Can you work these out from the model? Positions are in its coordinate system, mm. A direction names the side the tool comes from. Give positions to 0.01 mm unless a question says otherwise; leave off trailing zeros. Loops run counter-clockwise (first coordinate to the right, second up) from the corner with the lowest first, then second, coordinate; pieces in that order, holes last. Notation, with made-up numbers: (23.5, 59) -> (45.5, 59) arc R29 ccw to (45.5, 80) -> close; hole circle Ø4 at (86, 29). An arc over 180 degrees is marked (long way). Use CSV: the item, a comma, the result in double quotes.
from build123d import *

# Parameters (mm, degrees)
BOSS_EXTRUDE1_DEPTH      = 4.5
BOSS_EXTRUDE1_DEPTH_BACK = 4.5
SKETCH1_R                = 6.5
SKETCH1_R_2              = 4.5
SKETCH1_R_3              = 1.5
CUT_EXTRUDE1_DEPTH       = 3.5
CUT_EXTRUDE1_DEPTH_BACK  = 3.5
SKETCH1_3_R              = 6.5
SKETCH1_3_R_2            = 4.5


with BuildPart() as part:
    # Sketch1 → Boss-Extrude1 (new, two sides: drawn at the far end of the back side and taken through both)
    # profile 1 of 2: a face of its own
    with BuildSketch(Plane(origin=(0, 0, 0), x_dir=(0, 0, -1), z_dir=(1, 0, 0)).offset(-BOSS_EXTRUDE1_DEPTH_BACK)):
        Circle(SKETCH1_R)
        Circle(SKETCH1_R_2, mode=Mode.SUBTRACT)
    # profile 2 of 2: a face of its own
    with BuildSketch(Plane(origin=(0, 0, 0), x_dir=(0, 0, -1), z_dir=(1, 0, 0)).offset(-BOSS_EXTRUDE1_DEPTH_BACK)):
        Circle(SKETCH1_R_2)
        Circle(SKETCH1_R_3, mode=Mode.SUBTRACT)
    extrude(amount=BOSS_EXTRUDE1_DEPTH + BOSS_EXTRUDE1_DEPTH_BACK)

    # Sketch1_3 → Cut-Extrude1 (cut, two sides: drawn at the far end of the back side and taken through both)
    with BuildSketch(Plane(origin=(0, 0, 0), x_dir=(0, 0, -1), z_dir=(1, 0, 0)).offset(-CUT_EXTRUDE1_DEPTH_BACK)):
        Circle(SKETCH1_3_R)
        Circle(SKETCH1_3_R_2, mode=Mode.SUBTRACT)
    extrude(amount=CUT_EXTRUDE1_DEPTH + CUT_EXTRUDE1_DEPTH_BACK, mode=Mode.SUBTRACT)


solid = part.part
(1) We'd pull the mould along Z, two halves only. Please class faces 1 (the face through (-0.05, 4.46, 0.59)), 2 (the face through (-0.06, 0.07, 1.5)), 3 (the face through (4.5, 2, 0)): released by +Z, released by -Z, zero draft, split by the parting line, or undercut.
Answer sheet:
face 1,"split by the parting line"
face 2,"undercut"
face 3,"zero draft"
(2) Which directions (+Z, -Z, +X, -X, +Y, -Y) give clear straight access to the entire face, cutting with the end or side of a thin tool? Please do faces 4 (the face through (-3.5, 1.54, 4.42)), 5 (the face through (-4.007, -3.955, 5.158)).
Answer sheet:
face 4,"none"
face 5,"+X, -X"
(3) If I drill on L1, parallel to X at y = 5.25, z = 3.25; L2, parallel to Y at x = 1.5, z = 0; L3, parallel to Z at x = 1.75, y = -1, over which ranges is the centre line in solid material (lowest first)? Write a range as from..to.
Answer sheet:
L1,"x = -4.5..-3.5, 3.5..4.5"
L2,"y = -4.5..-1.5, 1.5..4.5"
L3,"z = -4.39..-1.12, 1.12..4.39"
(4) If we section it at C-C, the plane x = 3.75: Write out the boundary of the cut face in (y, z).
Answer sheet:
outline,"circle Ø13 at (0, 0); hole circle Ø3 at (0, 0)"
(5) If we section it at D-D, the plane y = 3.75: Write out the boundary of the cut face in (x, z), then the cut area to 3 significant figures.
Answer sheet:
outline,"(-4.5, -5.31) -> (-3.5, -5.31) -> (-3.5, -2.49) -> (3.5, -2.49) -> (3.5, -5.31) -> (4.5, -5.31) -> (4.5, 5.31) -> (3.5, 5.31) -> (3.5, 2.49) -> (-3.5, 2.49) -> (-3.5, 5.31) -> (-4.5, 5.31) -> close"
area,"56.1 mm2"
(6) Will these pins go through, and if not, where does the flat tip stop? pin 1 Ø1.5 at (x, y) = (-0.5, -1.5) entering from -Z; pin 2 Ø2.5 at (y, z) = (0, 0) entering from +X; pin 3 Ø1 at (x, z) = (-2, -1) entering from +Y; pin 4 Ø1.5 at (x, y) = (-2.5, -1) entering from +Z.
Answer sheet:
pin 1,"stops at z = -4.44"
pin 2,"passes through"
pin 3,"stops at y = 4.47"
pin 4,"stops at z = 4.49"
(7) If we section it at A-A, the plane z = 0: Write out the boundary of the cut face in (x, y), then the cut area to 3 significant figures.
Answer sheet:
outline,"(-4.5, -6.5) -> (-3.5, -6.5) -> (-3.5, -4.5) -> (3.5, -4.5) -> (3.5, -6.5) -> (4.5, -6.5) -> (4.5, -1.5) -> (-4.5, -1.5) -> close; (-4.5, 1.5) -> (4.5, 1.5) -> (4.5, 6.5) -> (3.5, 6.5) -> (3.5, 4.5) -> (-3.5, 4.5) -> (-3.5, 6.5) -> (-4.5, 6.5) -> close"
area,"62.0 mm2"
